Build history of the part. All positions in model axes, mm. A direction names the side the tool comes from. Coordinates: 2 decimals unless noted, no trailing zeros. Order: outer loops, then holes, each group sorted by start corner. A loop starts at its lowest first (then second) coordinate and runs counter-clockwise, first axis right, second up. Notation, with made-up numbers: (24, 28) - (46, 28) arc R6 cw to (46, 35) - close; hole circle Ø1 at (87.25, 48.25). An arc over 180 degrees is marked (long way). Return JSON: item names as keys, results as strings.
Autodesk Inventor part; units mm, degrees
ref_plane "YZ Plane" through (0, 0, 0) normal (1, 0, 0) x (0, 1, 0)
ref_plane "XZ Plane" through (0, 0, 0) normal (0, 1, 0) x (-1, 0, 0)
ref_plane "XY Plane" through (0, 0, 0) normal (0, 0, 1) x (1, 0, 0)
sketch "Sketch1" plane through (0, 0, 0) normal (0, 1, 0) x (-1, 0, 0)
  line L0 (-53.3048, 57.4444) -> (73.6952, 57.4444)
  line L1 (73.6952, 57.4444) -> (73.6952, -488.6556)
  line L2 (73.6952, -488.6556) -> (-53.3048, -488.6556)
  line L3 (-53.3048, -488.6556) -> (-53.3048, 57.4444)
  point P0 (0, 0)
  dimension "d0" = 127
  dimension "d1" = 546.1
extrude "Extrusion1" add sketch "Sketch1" along normal blind 111.76
sketch "Sketch2" plane through (0, 111.76, 0) normal (0, 1, 0) x (1, 0, 0)
  line L0 (-38.6432, 129.0678) -> (-48.2952, 129.0678)
  line L1 (-48.2952, 129.0678) -> (-48.2952, 206.0298)
  line L2 (-48.2952, 206.0298) -> (-38.6432, 206.0298)
  line L3 (-38.6432, 206.0298) -> (-38.6432, 129.0678)
  line L4 (53.3048, -57.4444) -> (53.3048, 488.6556)
  line L5 (-73.6952, 488.6556) -> (-73.6952, -57.4444)
  line L6 (-73.6952, -57.4444) -> (53.3048, -57.4444)
  point P0 (0, 0)
  dimension "d4" = 9.652
  dimension "d5" = 76.962
  dimension "d8" = 25.4
  dimension "d9" = 186.5122
extrude "Extrusion2" add sketch "Sketch2" along normal blind 79.375
sketch "Sketch3" plane through (-38.6432, 111.76, -129.0678) normal (1, 0, 0) x (0, 0, -1)
  line L0 (16.1079, 65.0185) -> (71.5479, 65.0185) construction
  line L1 (71.5479, 65.0185) -> (71.5479, 29.0665) construction
  line L2 (71.5479, 29.0665) -> (16.1079, 29.0665) construction
  line L3 (16.1079, 29.0665) -> (16.1079, 65.0185) construction
  point P0 (-129.0678, -111.76)
sketch "Sketch4" plane through (0, 0, 0) normal (0, -1, 0) x (1, 0, 0)
  line L0 (-19.5932, -155.9156) -> (158.2068, -155.9156)
  line L1 (158.2068, -155.9156) -> (158.2068, -98.7656)
  line L2 (158.2068, -98.7656) -> (-19.5932, -98.7656)
  line L3 (-19.5932, -98.7656) -> (-19.5932, -155.9156)
  line L4 (-73.6952, -488.6556) -> (53.3048, -488.6556)
  line L5 (-73.6952, 57.4444) -> (-73.6952, -488.6556)
  point P0 (0, 0)
  dimension "d13" = 332.74
  dimension "d14" = 57.15
  dimension "d15" = 54.102
  dimension "d16" = 177.8
extrude "Extrusion3" add sketch "Sketch4" along normal blind 57.15
sketch "Sketch5" plane through (158.2068, 0, -155.9156) normal (0, 0, -1) x (-1, 0, 0)
  line L0 (25.6026, -7.1293) -> (89.7659, -7.1293) construction
  line L1 (89.7659, -7.1293) -> (89.7659, -41.3497) construction
  line L2 (89.7659, -41.3497) -> (25.6026, -41.3497) construction
  line L3 (25.6026, -41.3497) -> (25.6026, -7.1293) construction
  point P0 (158.2068, 0)
properties part number "CLB_056_4StagePlaceholder"
1. Probe L1, parallel to Z at x = 63, y = -34; L2, parallel to X at y = 34.5, z = -405.5; L3, parallel to Y at x = 0, z = -2. List the from-to ranges inside material, lowest first.
Check values:
{"L1": "-155.92 to -98.77", "L2": "-73.7 to 53.3", "L3": "0 to 111.76"}
2. Cut at C-C on z = -367. Give the cut face in (x, y).
Check values:
{"outline": "(-73.7, 0) - (53.3, 0) - (53.3, 111.76) - (-73.7, 111.76) - close"}
3. Cut at B-B on y = 138.5. Give the cut face in (x, z).
Check values:
{"outline": "(-48.3, -206.03) - (-38.64, -206.03) - (-38.64, -129.07) - (-48.3, -129.07) - close"}
4. Cut at A-A on x = 26.5. Give the cut face in (y, z), plus the area to 3 significant figures.
Check values:
{"outline": "(-57.15, -155.92) - (0, -155.92) - (0, -488.66) - (111.76, -488.66) - (111.76, 57.44) - (0, 57.44) - (0, -98.77) - (-57.15, -98.77) - close", "area": "64,300 mm²"}
5. Drop flat-ended pins along their axis: pin 1 (5 mm diameter, centred on x = 6, z = -251, fed in from +Y); pin 2 (5 mm diameter, centred on x = -43, y = 152, fed in from +Z); pin 3 (23 mm diameter, centred on y = 171, z = -163, fed in from +X). Give the stop position or say it passes through.
Check values:
{"pin 1": "y = 111.76", "pin 2": "z = -129.07", "pin 3": "x = -38.64"}
6. Tool access for faces 1 (the flat face through (71, -28, -98.766)), 2 (the flat face through (-44, 151, -206.03)), 3 (the flat face through (-48.295, 151, -167)), 4 (the flat face through (105, 0, -127)): list every direction of +Z, -Z, +X, -X, +Y, -Y with a clear straight run to the whole face (end or side of a thin tool).
Check values:
{"face 1": "+Z, +X, -X, -Y", "face 2": "-Z, +X, -X, +Y", "face 3": "+Z, -Z, -X, +Y", "face 4": "+Z, -Z, +X, +Y"}
